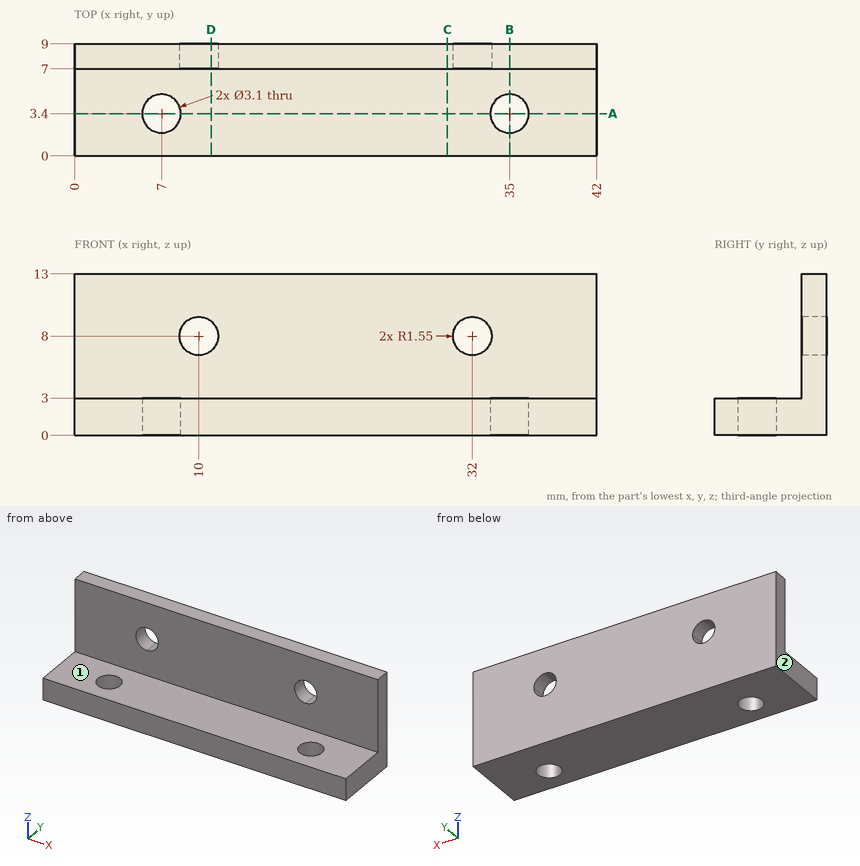
Could you check a few things on this drawing? It's one solid part, dimensions in mm from its lowest x, y, z. A direction names the side the tool comes from. Round coordinates to 2 decimals unless told otherwise and drop trailing zeros. Write each loop counter-clockwise with the first axis right and the second up, starting at its lowest first coordinate (ties: lowest second). Pieces come first, ordered by that corner, then holes. Notation, with made-up numbers: M 45.25,32.5 L 83.25,32.5 A21 ccw 83.25,64.5 Z; hole C 84,-36.5 d7. An arc over 180 degrees is marked long. Answer as CSV lines item,"result". Start each with the question number.
1. I'm going to push flat-ended pins straight in: pin 1 Ø5 at (x, y) = (28, 3.5) entering from +Z; pin 2 Ø3 at (x, z) = (20.5, 6.5) entering from -Y. Where does each tip first touch, or does it pass through?
2. Suppose I cut it at D-D on x = 11. Write out the boundary of the cut face in (y, z).
3. Suppose I cut it at B-B on x = 35. Write out the boundary of the cut face in (y, z).
4. I need wall thicknesses on probe 1 along Y at (x, z) = (35, 1.9); probe 2 along Z at (x, y) = (22.5, 6.75); probe 3 along Y at (x, z) = (27.5, 10.75). Which ranges of each line are inside material? Lowest first, please.
5. On a 3-axis mill with a long thin cutter (end or side, diameter ignored), from which of +Z, -Z, +X, -X, +Y, -Y can I reach the whole of each face in a straight line? I mean the marked faces 1 and 2. Say none if no direction works.
6. Suppose I cut it at A-A on y = 3.4. Write out the boundary of the cut face in (x, z).
7. Suppose I cut it at C-C on x = 30. Write out the boundary of the cut face in (y, z), then the cut area to 3 significant figures.
Check result:
1,pin 1,"stops at z = 3"
1,pin 2,"stops at y = 7"
2,outline,"M 0,0 L 9,0 L 9,6.82 L 7,6.82 L 7,3 L 0,3 Z; M 7,9.18 L 9,9.18 L 9,13 L 7,13 Z"
3,outline,"M 0,0 L 1.85,0 L 1.85,3 L 0,3 Z; M 4.95,0 L 9,0 L 9,13 L 7,13 L 7,3 L 4.95,3 Z"
4,probe 1,"y = 0 to 1.85, 4.95 to 9"
4,probe 2,"z = 0 to 3"
4,probe 3,"y = 7 to 9"
5,face 1,"+Z, +X, -X, -Y"
5,face 2,"+Z, -Z, -X, +Y, -Y"
6,outline,"M 0,0 L 5.45,0 L 5.45,3 L 0,3 Z; M 8.55,0 L 33.45,0 L 33.45,3 L 8.55,3 Z; M 36.55,0 L 42,0 L 42,3 L 36.55,3 Z"
7,outline,"M 0,0 L 9,0 L 9,13 L 7,13 L 7,3 L 0,3 Z"
7,area,"47.0 mm2"
